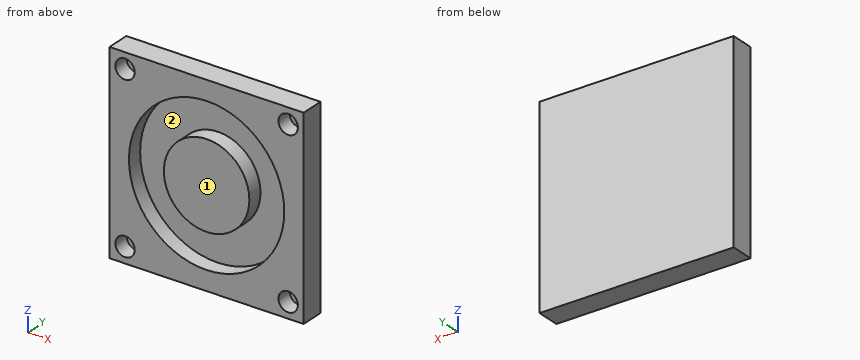
from build123d import *

# Parameters (mm, degrees)
SKETCH1_W           = 25
SKETCH1_H           = 25
BOSS_EXTRUDE1_DEPTH = 3
CAVITY1_OUTLINE_R   = 10
CAVITY1_OUTLINE_R_2 = 5.5
CAVITY1_DEPTH       = 2
SKETCH2_R           = 1.25
CUT_EXTRUDE1_DEPTH  = 2


# Read off the part's stored shape, not the designer's step: Cavity1
with BuildPart() as part:
    # Sketch1 → Boss-Extrude1 (new body)
    with BuildSketch(Plane(origin=(0, 0, 0), x_dir=(1, 0, 0), z_dir=(0, 1, 0))):
        Rectangle(SKETCH1_W, SKETCH1_H)
    extrude(amount=BOSS_EXTRUDE1_DEPTH)

    # Cavity1 outline → Cavity1 (cut)
    with BuildSketch(Plane(origin=(0, 0, 0), x_dir=(1, 0, 0), z_dir=(0, 1, 0))):
        Circle(CAVITY1_OUTLINE_R)
        Circle(CAVITY1_OUTLINE_R_2, mode=Mode.SUBTRACT)
    extrude(amount=CAVITY1_DEPTH, mode=Mode.SUBTRACT)

    # Sketch2 → Cut-Extrude1 (cut)
    with BuildSketch(Plane.XZ):
        with Locations(Location((-10.5, 10.5, 0), (0, 0, 270))):
            Circle(SKETCH2_R)
        with Locations(Location((10.5, 10.5, 0), (0, 0, 270))):
            Circle(SKETCH2_R)
        with Locations(Location((10.5, -10.5, 0), (0, 0, 270))):
            Circle(SKETCH2_R)
        with Locations(Location((-10.5, -10.5, 0), (0, 0, 270))):
            Circle(SKETCH2_R)
    extrude(amount=-CUT_EXTRUDE1_DEPTH, mode=Mode.SUBTRACT)


solid = part.part
Design review of the part built by this model. Coordinates are the model's own, in mm. Face numbers are marked on the shaded views. Round coordinates to 2 decimals unless told otherwise and drop trailing zeros. Loops run counter-clockwise (first coordinate to the right, second up) from the corner with the lowest first, then second, coordinate; pieces in that order, holes last. Notation, with made-up numbers: (17.25, 5.25) - (70.25, 5.25) arc R10 cw to (70.25, 23.25) - close; hole circle Ø10 at (-23.75, 87). An arc over 180 degrees is marked (long way). One line per item, written item: value. Start each with the question number.
1) Consider section A-A on y = 1. Give the boundary of the cut face in (x, z), then the cut area to 3 significant figures.
2) To check wall thickness, follow L1, parallel to X at y = 1.05, z = 0; L2, parallel to X at y = 0.5, z = 10.5; L3, parallel to Z at x = -0.25, y = 1.5. State the ranges of each line that lie inside material, in increasing order. Write a range as from..to.
3) Insertion check: pin 1 Ø0.8 at (x, z) = (-10.5, 10) entering from -Y; pin 2 Ø3 at (x, z) = (10, -10) entering from -Y. Each pin has a flat end and moves straight along its axis. Give the tip position at first contact, or say it passes through.
4) Consider section D-D on x = -6.75. Give the boundary of the cut face in (y, z).
5) Consider section C-C on x = -10.5. Give the boundary of the cut face in (y, z), then the cut area to 3 significant figures.
6) Draft analysis for pull direction Z (two halves, no side actions). For the marked faces 1 and 2, state which applies: +Z half, -Z half, draft (parallel to the pull), parting line (faces both ways), or undercut.
7) Consider section B-B on z = 0. Give the boundary of the cut face in (x, y), then the cut area to 3 significant figures.
Reported:
1. outline: (-12.5, -12.5) - (12.5, -12.5) - (12.5, 12.5) - (-12.5, 12.5) - close; circle Ø11 at (0, 0); hole circle Ø2.5 at (-10.5, -10.5); hole circle Ø2.5 at (-10.5, 10.5); hole circle Ø20 at (0, 0); hole circle Ø2.5 at (10.5, -10.5); hole circle Ø2.5 at (10.5, 10.5)
1. area: 386 mm^2
2. L1: x = -12.5..-10, -5.5..5.5, 10..12.5
2. L2: x = -12.5..-11.75, -9.25..9.25, 11.75..12.5
2. L3: z = -12.5..-10, -5.49..5.49, 10..12.5
3. pin 1: stops at y = 2
3. pin 2: stops at y = 0
4. outline: (0, -12.5) - (3, -12.5) - (3, 12.5) - (0, 12.5) - (0, 7.38) - (2, 7.38) - (2, -7.38) - (0, -7.38) - close
5. outline: (0, -12.5) - (3, -12.5) - (3, 12.5) - (0, 12.5) - (0, 11.75) - (2, 11.75) - (2, 9.25) - (0, 9.25) - (0, -9.25) - (2, -9.25) - (2, -11.75) - (0, -11.75) - close
5. area: 65.0 mm^2
6. face 1: draft
6. face 2: undercut
7. outline: (-12.5, 0) - (-10, 0) - (-10, 2) - (-5.5, 2) - (-5.5, 0) - (5.5, 0) - (5.5, 2) - (10, 2) - (10, 0) - (12.5, 0) - (12.5, 3) - (-12.5, 3) - close
7. area: 57.0 mm^2
